Could you check a few things on this model? Use its own coordinates, in mm. Face numbers are marked on the shaded views. Give positions to 0.01 mm unless a question says otherwise; leave off trailing zeros. Order: outer loops, then holes, each group sorted by start corner. A loop starts at its lowest first (then second) coordinate and runs counter-clockwise, first axis right, second up. Notation, with made-up numbers: M 40.5,10.25 L 69.5,10.25 A10 ccw 69.5,20.25 Z; hole C -36,48 d7. An arc over 180 degrees is marked long. Answer in a Markdown table with one row per item. Add a question column.
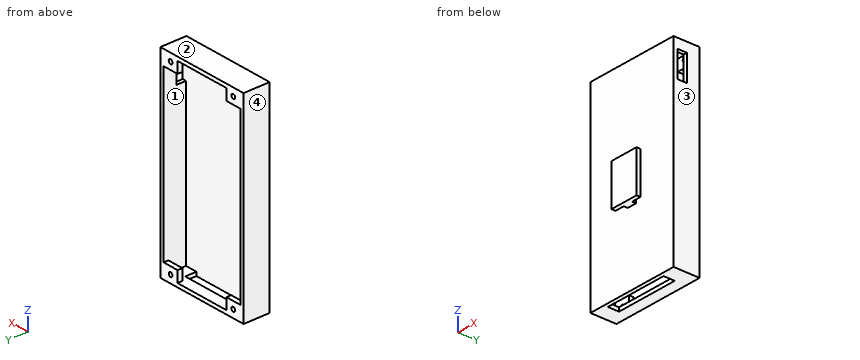
```python
from build123d import *

# Parameters (mm, degrees)
SKETCH1_W               = 75.85
SKETCH1_H               = 158.4
BOSS_EXTRUDE1_DEPTH     = 3
SKETCH2_W               = 75.85
SKETCH2_H               = 158.4
SKETCH2_W_2             = 69.85
SKETCH2_H_2             = 152.4
BOSS_EXTRUDE2_DEPTH     = 17.78
SKETCH3_W               = 12.7
SKETCH3_H               = 8.89
BOSS_EXTRUDE3_DEPTH     = 3.81
SKETCH7_W               = 50.8
SKETCH7_H               = 42.7
BOSS_EXTRUDE4_DEPTH     = 6.35
CUT_EXTRUDE2_DEPTH      = 110.455089078
CUT_EXTRUDE2_DEPTH_BACK = 110.455089078
CUT_EXTRUDE3_START      = -6.35
SKETCH9_W               = 22.86
SKETCH9_H               = 9.7
CUT_EXTRUDE3_DEPTH      = 6.35
CUT_EXTRUDE4_REACH      = 93.907
SKETCH4_R               = 1.7
SKETCH4_R_2             = 1.72
CUT_EXTRUDE5_REACH      = 166.197
SKETCH10_W              = 50.8
SKETCH10_H              = 8.89
CUT_EXTRUDE6_REACH      = 113.614
SKETCH11_W              = 20.828
SKETCH11_H              = 7.62


with BuildPart() as part:
    # Sketch1 → Boss-Extrude1 (new body)
    with BuildSketch(Plane(origin=(0, 0, 0), x_dir=(1, 0, 0), z_dir=(0, 1, 0))):
        Rectangle(SKETCH1_W, SKETCH1_H)
    extrude(amount=BOSS_EXTRUDE1_DEPTH)

    # Sketch2 → Boss-Extrude2 (add)
    with BuildSketch(Plane(origin=(0, 3, 0), x_dir=(1, 0, 0), z_dir=(0, 1, 0))):
        Rectangle(SKETCH2_W, SKETCH2_H)
        Rectangle(SKETCH2_W_2, SKETCH2_H_2, mode=Mode.SUBTRACT)
    extrude(amount=BOSS_EXTRUDE2_DEPTH)

    # Sketch3 → Boss-Extrude3 (add)
    with BuildSketch(Plane(origin=(0, 20.78, 0), x_dir=(1, 0, 0), z_dir=(0, 1, 0))):
        with Locations((-28.575, 71.755)):
            Rectangle(SKETCH3_W, SKETCH3_H)
        with Locations((-28.575, -71.755)):
            Rectangle(SKETCH3_W, SKETCH3_H)
        with Locations((28.575, 71.755)):
            Rectangle(SKETCH3_W, SKETCH3_H)
        with Locations((28.575, -71.755)):
            Rectangle(SKETCH3_W, SKETCH3_H)
    extrude(amount=-BOSS_EXTRUDE3_DEPTH)

    # Sketch7 → Boss-Extrude4 (add)
    with BuildSketch(Plane.XZ):
        Rectangle(SKETCH7_W, SKETCH7_H)
    extrude(amount=BOSS_EXTRUDE4_DEPTH)

    # Sketch8 → Cut-Extrude2 (cut, two sides: drawn at the far end of the back side and taken through both)
    with BuildSketch(Plane.XY.offset(21.35).offset(-CUT_EXTRUDE2_DEPTH_BACK)):
        Polygon((-3.81, -3.175), (-3.81, 0), (-25.4, 0), (-25.4, -6.35), (-11.43, -6.35), (-11.43, -3.175), align=None)
        Polygon((25.4, 0), (3.81, 0), (3.81, -3.175), (11.43, -3.175), (11.43, -6.35), (25.4, -6.35), align=None)
    extrude(amount=CUT_EXTRUDE2_DEPTH + CUT_EXTRUDE2_DEPTH_BACK, mode=Mode.SUBTRACT)

    # Sketch9 → Cut-Extrude3 (cut)
    with BuildSketch(Plane.XZ.offset(6.35).offset(CUT_EXTRUDE3_START)):
        with Locations((0, 16.5)):
            Rectangle(SKETCH9_W, SKETCH9_H)
    extrude(amount=CUT_EXTRUDE3_DEPTH, mode=Mode.SUBTRACT)

    # Sketch4 → Cut-Extrude4 (cut, up to next)
    with BuildSketch(Plane(origin=(0, 20.78, 0), x_dir=(1, 0, 0), z_dir=(0, 1, 0)), mode=Mode.PRIVATE) as cut_extrude4_sk1:
        with Locations(Location((-28.575, 73.025, 0), (0, 0, 270))):
            Circle(SKETCH4_R)
    cut_extrude4_tool1 = extrude(cut_extrude4_sk1.sketch, amount=-CUT_EXTRUDE4_REACH, mode=Mode.PRIVATE) & part.part
    # Sketch4 → Cut-Extrude4 (cut, up to next)
    with BuildSketch(Plane(origin=(0, 20.78, 0), x_dir=(1, 0, 0), z_dir=(0, 1, 0)), mode=Mode.PRIVATE) as cut_extrude4_sk2:
        with Locations(Location((28.575, 73.025, 0), (0, 0, 270))):
            Circle(SKETCH4_R)
    cut_extrude4_tool2 = extrude(cut_extrude4_sk2.sketch, amount=-CUT_EXTRUDE4_REACH, mode=Mode.PRIVATE) & part.part
    # Sketch4 → Cut-Extrude4 (cut, up to next)
    with BuildSketch(Plane(origin=(0, 20.78, 0), x_dir=(1, 0, 0), z_dir=(0, 1, 0)), mode=Mode.PRIVATE) as cut_extrude4_sk3:
        with Locations(Location((28.575, -73.025, 0), (0, 0, 270))):
            Circle(SKETCH4_R_2)
    cut_extrude4_tool3 = extrude(cut_extrude4_sk3.sketch, amount=-CUT_EXTRUDE4_REACH, mode=Mode.PRIVATE) & part.part
    # Sketch4 → Cut-Extrude4 (cut, up to next)
    with BuildSketch(Plane(origin=(0, 20.78, 0), x_dir=(1, 0, 0), z_dir=(0, 1, 0)), mode=Mode.PRIVATE) as cut_extrude4_sk4:
        with Locations(Location((-28.575, -73.025, 0), (0, 0, 270))):
            Circle(SKETCH4_R)
    cut_extrude4_tool4 = extrude(cut_extrude4_sk4.sketch, amount=-CUT_EXTRUDE4_REACH, mode=Mode.PRIVATE) & part.part
    add(cut_extrude4_tool1.solids().sort_by_distance((-28.575, 20.78, -73.025))[0], mode=Mode.SUBTRACT)
    add(cut_extrude4_tool2.solids().sort_by_distance((28.575, 20.78, -73.025))[0], mode=Mode.SUBTRACT)
    add(cut_extrude4_tool3.solids().sort_by_distance((28.575, 20.78, 73.025))[0], mode=Mode.SUBTRACT)
    add(cut_extrude4_tool4.solids().sort_by_distance((-28.575, 20.78, 73.025))[0], mode=Mode.SUBTRACT)

    # Sketch10 → Cut-Extrude5 (cut, up to next)
    with BuildSketch(Plane(origin=(0, 0, -79.2), x_dir=(-1, 0, 0), z_dir=(0, 0, -1)), mode=Mode.PRIVATE) as cut_extrude5_sk1:
        with Locations((0, 7.445)):
            Rectangle(SKETCH10_W, SKETCH10_H)
    cut_extrude5_tool1 = extrude(cut_extrude5_sk1.sketch, amount=-CUT_EXTRUDE5_REACH, mode=Mode.PRIVATE) & part.part
    add(cut_extrude5_tool1.solids().sort_by_distance((0, 7.445, -79.2))[0], mode=Mode.SUBTRACT)

    # Sketch11 → Cut-Extrude6 (cut, up to next)
    with BuildSketch(Plane(origin=(37.925, 0, 0), x_dir=(0, 0, -1), z_dir=(1, 0, 0)), mode=Mode.PRIVATE) as cut_extrude6_sk1:
        with Locations((-61.166, 6.81)):
            Rectangle(SKETCH11_W, SKETCH11_H)
    cut_extrude6_tool1 = extrude(cut_extrude6_sk1.sketch, amount=-CUT_EXTRUDE6_REACH, mode=Mode.PRIVATE) & part.part
    add(cut_extrude6_tool1.solids().sort_by_distance((37.925, 6.81, 61.166))[0], mode=Mode.SUBTRACT)


solid = part.part
```
1. Suppose I cut it at A-A on y = 13.5. List the corners of the cut face in (x, z) for me (3 decimals), plus the area to 3 significant figures.
2. If I drill on line 1 along Y through (x, z) = (-6.5, -2) (3 decimals); line 2 along X through (y, z) = (3.75, -43) (3 decimals); line 3 along Y through (x, z) = (-29, 71), over which ranges is the centre line in solid material (lowest first)? Write a range as [from, to].
3. Will these pins go through, and if not, where does the flat tip stop? P1, Ø0.9, axis at x = 36, z = 56, coming from the -Y side; P2, Ø6, axis at x = 21.5, z = -27, coming from the +Y side; P3, Ø3, axis at x = -3.5, y = -3.5, coming from the +Z side; P4, Ø12, axis at y = -0.5, z = -62, coming from the +X side (3 decimals).
4. Suppose I cut it at B-B on x = 19.5. List the corners of the cut face in (y, z) for me, plus the area to 3 significant figures.
5. Suppose I cut it at D-D on y = 4.75. List the corners of the cut face in (x, z) for me (3 decimals), plus the area to 3 significant figures.
6. Thinking about a two-plate mould opening in X: for the marked faces 1, 2, 3 and 4, which applies, pulls with the +X half, pulls with the -X half, needs draft (parallel to the pull), parting line crosses it, or undercut?
7. Suppose I cut it at C-C on x = -6. List the corners of the cut face in (y, z) for me (3 decimals).
Findings below:
| question | item | result |
|---|---|---|
| 1 | outline | M -37.925,-79.2 L 37.925,-79.2 L 37.925,79.2 L -37.925,79.2 Z; hole M -34.925,-76.2 L 34.925,-76.2 L 34.925,76.2 L -34.925,76.2 Z |
| 1 | area | 1,370 mm2 |
| 2 | line 1 | [-6.35, -3.175], [0, 3] |
| 2 | line 2 | [-37.925, -34.925], [34.925, 37.925] |
| 2 | line 3 | [0, 3], [16.97, 20.78] |
| 3 | P1 | y = 0 |
| 3 | P2 | y = 3 |
| 3 | P3 | z = 11.65 |
| 3 | P4 | x = 37.925 |
| 4 | outline | M 0,-79.2 L 3,-79.2 L 3,76.2 L 20.78,76.2 L 20.78,79.2 L 0,79.2 Z; M 11.89,-79.2 L 20.78,-79.2 L 20.78,-76.2 L 11.89,-76.2 Z |
| 4 | area | 555 mm2 |
| 5 | outline | M -37.925,-79.2 L -25.4,-79.2 L -25.4,-76.2 L -34.925,-76.2 L -34.925,76.2 L 34.925,76.2 L 34.925,71.58 L 37.925,71.58 L 37.925,79.2 L -37.925,79.2 Z; M 25.4,-79.2 L 37.925,-79.2 L 37.925,50.752 L 34.925,50.752 L 34.925,-76.2 L 25.4,-76.2 Z |
| 5 | area | 1,150 mm2 |
| 6 | face 1 | undercut |
| 6 | face 2 | needs draft |
| 6 | face 3 | pulls with the +X half |
| 6 | face 4 | pulls with the -X half |
| 7 | outline | M -6.35,-21.35 L -3.175,-21.35 L -3.175,11.65 L -6.35,11.65 Z; M 0,-79.2 L 3,-79.2 L 3,76.2 L 20.78,76.2 L 20.78,79.2 L 0,79.2 Z; M 11.89,-79.2 L 20.78,-79.2 L 20.78,-76.2 L 11.89,-76.2 Z |
